Here's how the part is built. I have some questions about the finished solid (model axes, mm). Face numbers are marked on the shaded views. A direction names the side the tool comes from. Give positions to 0.01 mm unless a question says otherwise; leave off trailing zeros. Order: outer loops, then holes, each group sorted by start corner. A loop starts at its lowest first (then second) coordinate and runs counter-clockwise, first axis right, second up. Notation, with made-up numbers: (-27, -39) -> (-20, -39) arc R9 ccw to (-20, -33) -> close; hole circle Ø5 at (30.25, 36). An arc over 180 degrees is marked (long way). Write each question's results on one line, items separated by ' | '. Start each with the question number.
Q1. Imagine slicing it at B-B, the plane z = 4. Please give me the cut outline in (x, y), then the cut area to 3 significant figures.
Q2. Imagine slicing it at A-A, the plane x = -3. Please give me the cut outline in (y, z), then the cut area to 3 significant figures.
Q3. Imagine slicing it at D-D, the plane z = 3. Please give me the cut outline in (x, y).
Q4. Thinking about a two-plate mould opening in Y: for the marked faces 1, 2 and 3, which applies, pulls with the +Y half, pulls with the -Y half, needs draft (parallel to the pull), parting line crosses it, or undercut?
Q5. I need wall thicknesses on line 1 along Y through (x, z) = (-3.3, 4); line 2 along Y through (x, z) = (-2.05, 4); line 3 along X through (y, z) = (-8.5, 3.5). Which ranges of each line are inside material? Lowest first, please. Write a range as [from, to].
Q6. I'm going to push flat-ended pins straight in: pin 1 (0.8 mm diameter, centred on x = -5, z = 2.5, fed in from +Y); pin 2 (4 mm diameter, centred on y = -5.5, z = 1, fed in from +X); pin 3 (1 mm diameter, centred on y = -10, z = 2, fed in from -X); pin 4 (3 mm diameter, centred on y = -5, z = 3, fed in from -X). Where does each tip first touch, or does it pass through?
Q7. Imagine slicing it at C-C, the plane z = 7.75. Please give me the cut outline in (x, y), then the cut area to 3 significant figures.
Q8. For the marked faces 4 and 5, which set-ups out of +Z, -Z, +X, -X, +Y, -Y let a thin tool reach every point of the face, with its end or its side?
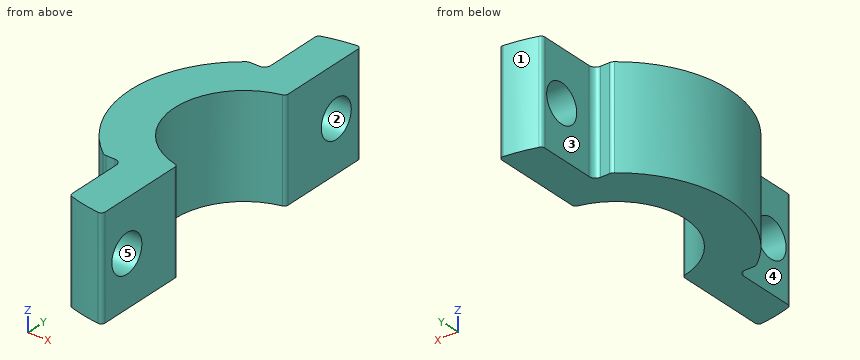
```python
from build123d import *

# Parameters (mm, degrees)
ESQUISSE1_R             = 13
ESQUISSE1_R_2           = 5.5
BOSS_EXTRU_1_DEPTH      = 8
ESQUISSE2_W             = 32.31004566
ESQUISSE2_H             = 49.818141682
ENL_V_MAT_EXTRU_1_DEPTH = 8
ESQUISSE3_R             = 1.5
ENL_V_MAT_EXTRU_2_DEPTH = 8
ESQUISSE4_W             = 24.87123002
ESQUISSE4_H             = 13.833010023
ESQUISSE4_W_2           = 23.432073676
ESQUISSE4_H_2           = 10.309386407
ENL_V_MAT_EXTRU_3_DEPTH = 8
ENL_V_MAT_EXTRU_4_DEPTH = 8
CONG_1_R                = 0.5
CONG_3_R                = 0.3
CONG_4_R                = 0.5


with BuildPart() as part:
    # Esquisse1 → Boss.-Extru.1 (new body)
    with BuildSketch(Plane.XY):
        Circle(ESQUISSE1_R)
        Circle(ESQUISSE1_R_2, mode=Mode.SUBTRACT)
    extrude(amount=BOSS_EXTRU_1_DEPTH)

    # Esquisse2 → Enlèv. mat.-Extru.1 (cut)
    with BuildSketch(Plane.XY.offset(8)):
        with Locations((15.15502283, -0.665904075)):
            Rectangle(ESQUISSE2_W, ESQUISSE2_H)
    extrude(amount=-ENL_V_MAT_EXTRU_1_DEPTH, mode=Mode.SUBTRACT)

    # Esquisse3 → Enlèv. mat.-Extru.2 (cut)
    with BuildSketch(Plane(origin=(-1, 0, 0), x_dir=(0, 0, -1), z_dir=(1, 0, 0))):
        with Locations((-4, 10.461481397)):
            Circle(ESQUISSE3_R)
        with Locations((-4, -10.461481397)):
            Circle(ESQUISSE3_R)
    extrude(amount=-ENL_V_MAT_EXTRU_2_DEPTH, mode=Mode.SUBTRACT)

    # Esquisse4 → Enlèv. mat.-Extru.3 (cut)
    with BuildSketch(Plane.XY.offset(8)):
        with Locations((-16.43561501, 14.127986408)):
            Rectangle(ESQUISSE4_W, ESQUISSE4_H)
        with Locations((-15.716036838, -12.366174601)):
            Rectangle(ESQUISSE4_W_2, ESQUISSE4_H_2)
    extrude(amount=-ENL_V_MAT_EXTRU_3_DEPTH, mode=Mode.SUBTRACT)

    # Esquisse6 → Enlèv. mat.-Extru.4 (cut)
    with BuildSketch(Plane.XY.offset(8)):
        with BuildLine():
            Line((-15.190239973, -9.672332462), (-4.630180203, -7.717605282))
            ThreePointArc((-4.630180203, -7.717605282), (-8.999645968, -0.079827604), (-4.766352493, 7.63425726))
            Line((-4.766352493, 7.63425726), (-11.634503641, 11.269457117))
            ThreePointArc((-11.634503641, 11.269457117), (-18.222154917, 1.615222264), (-15.190239973, -9.672332462))
        make_face()
    extrude(amount=-ENL_V_MAT_EXTRU_4_DEPTH, mode=Mode.SUBTRACT)

    # Congé1
    cong_1_edges = [part.edges().sort_by_distance(p)[0] for p in [
        (-4, 7.211481397, 4),
        (-4, -7.211481397, 4),
    ]]
    fillet(cong_1_edges, radius=CONG_1_R)

    # Congé3
    cong_3_edges = [part.edges().sort_by_distance(p)[0] for p in [
        (-1, -5.408326913, 4),
        (-1, 5.408326913, 4),
        (-1, 12.961481397, 4),
        (-1, -12.961481397, 4),
        (-4, 12.369316877, 4),
        (-4, -12.369316877, 4),
    ]]
    fillet(cong_3_edges, radius=CONG_3_R)

    # Congé4
    cong_4_edges = [part.edges().sort_by_distance(p)[0] for p in [
        (-5.384657469, 7.211481397, 4),
        (-5.384657469, -7.211481397, 4),
    ]]
    fillet(cong_4_edges, radius=CONG_4_R)


solid = part.part
```
Geometry check:
1) outline: (-5.52, -7.11) arc R0.5 ccw to (-5.22, -7.21) -> (-4.5, -7.21) arc R0.5 cw to (-4, -7.71) -> (-4, -8.96) -> (-1, -8.96) -> (-1, -5.65) arc R0.3 ccw to (-1.23, -5.36) arc R5.5 cw to (-1.23, 5.36) arc R0.3 ccw to (-1, 5.65) -> (-1, 8.96) -> (-4, 8.96) -> (-4, 7.71) arc R0.5 cw to (-4.5, 7.21) -> (-5.22, 7.21) arc R0.5 ccw to (-5.52, 7.11) arc R9 ccw to start; (-4, -12.15) arc R0.3 ccw to (-3.79, -12.44) arc R13 ccw to (-1.33, -12.93) arc R0.3 ccw to (-1, -12.63) -> (-1, -11.96) -> (-4, -11.96) -> close; (-4, 11.96) -> (-1, 11.96) -> (-1, 12.63) arc R0.3 ccw to (-1.33, 12.93) arc R13 ccw to (-3.79, 12.44) arc R0.3 ccw to (-4, 12.15) -> close | area: 78.2 mm²
2) outline: (-12.65, 0) -> (-4.61, 0) -> (-4.61, 8) -> (-12.65, 8) -> close; (4.61, 0) -> (12.65, 0) -> (12.65, 8) -> (4.61, 8) -> close; hole circle Ø3 at (-10.46, 4); hole circle Ø3 at (10.46, 4) | area: 114 mm²
3) outline: (-5.52, -7.11) arc R0.5 ccw to (-5.22, -7.21) -> (-4.5, -7.21) arc R0.5 cw to (-4, -7.71) -> (-4, -9.34) -> (-1, -9.34) -> (-1, -5.65) arc R0.3 ccw to (-1.23, -5.36) arc R5.5 cw to (-1.23, 5.36) arc R0.3 ccw to (-1, 5.65) -> (-1, 9.34) -> (-4, 9.34) -> (-4, 7.71) arc R0.5 cw to (-4.5, 7.21) -> (-5.22, 7.21) arc R0.5 ccw to (-5.52, 7.11) arc R9 ccw to start; (-4, -12.15) arc R0.3 ccw to (-3.79, -12.44) arc R13 ccw to (-1.33, -12.93) arc R0.3 ccw to (-1, -12.63) -> (-1, -11.58) -> (-4, -11.58) -> close; (-4, 11.58) -> (-1, 11.58) -> (-1, 12.63) arc R0.3 ccw to (-1.33, 12.93) arc R13 ccw to (-3.79, 12.44) arc R0.3 ccw to (-4, 12.15) -> close
4) face 1: pulls with the +Y half | face 2: undercut | face 3: needs draft
5) line 1: [-12.57, -11.96], [-8.96, -4.4], [4.4, 8.96], [11.96, 12.57] | line 2: [-12.84, -11.96], [-8.96, -5.1], [5.1, 8.96], [11.96, 12.84] | line 3: [-4, -1]
6) pin 1: y = 7.21 | pin 2: x = -1 | pin 3: x = -4 | pin 4: x = -8.29
7) outline: (-5.52, -7.11) arc R0.5 ccw to (-5.22, -7.21) -> (-4.5, -7.21) arc R0.5 cw to (-4, -7.71) -> (-4, -12.15) arc R0.3 ccw to (-3.79, -12.44) arc R13 ccw to (-1.33, -12.93) arc R0.3 ccw to (-1, -12.63) -> (-1, -5.65) arc R0.3 ccw to (-1.23, -5.36) arc R5.5 cw to (-1.23, 5.36) arc R0.3 ccw to (-1, 5.65) -> (-1, 12.63) arc R0.3 ccw to (-1.33, 12.93) arc R13 ccw to (-3.79, 12.44) arc R0.3 ccw to (-4, 12.15) -> (-4, 7.71) arc R0.5 cw to (-4.5, 7.21) -> (-5.22, 7.21) arc R0.5 ccw to (-5.52, 7.11) arc R9 ccw to start | area: 96.2 mm²
8) face 4: +Z, -Z, -X, -Y | face 5: +X, -X
